Autodesk Inventor part; units mm, degrees
ref_plane "YZ Plane" through (0, 0, 0) normal (1, 0, 0) x (0, 1, 0)
ref_plane "XZ Plane" through (0, 0, 0) normal (0, 1, 0) x (-1, 0, 0)
ref_plane "XY Plane" through (0, 0, 0) normal (0, 0, 1) x (1, 0, 0)
sketch "スケッチ1" plane through (0, 0, 0) normal (0, 0, 1) x (1, 0, 0)
  line L0 (0, 0) -> (-26, 0)
  line L1 (0, 0) -> (-13, -73.8647)
  line L2 (-13, -73.8647) -> (-26, 0)
  dimension "d0" = 26
  dimension "d1" = 75
extrude "押し出し1" add sketch "スケッチ1" along normal mid plane 18
sketch "スケッチ2" plane through (0, 0, 9) normal (0, 0, 1) x (1, 0, 0)
  line L0 (-26, 0) -> (0, 0)
  line L1 (-2, 0) -> (-24, 0)
  line L2 (-2, 0) -> (-12.9991, -62.5063)
  line L3 (-2, 0) -> (61.4667, 0) construction
  line L4 (-12.9991, -62.5063) -> (-24, 0)
  line L5 (-13, -73.8647) -> (-26, 0)
  point P0 (-15.5606, -59.3154)
  dimension "d5" = 22
  dimension "d6" = 99.98
extrude "押し出し2" cut sketch "スケッチ2" against normal blind 20
fillet "フィレット2" radius 1 1 edges at (-12.9991, -62.5063, 0)
fillet "フィレット3" radius 2.6 1 edges at (-13, -73.8647, 0)
sketch "スケッチ3" plane through (0, 0, 9) normal (0, 0, 1) x (1, 0, 0)
  line L0 (-12.0143, -56.9099) -> (-2, 0)
  line L1 (-2.7039, -4) -> (-23.296, -4)
  line L2 (-13.984, -56.9099) -> (-24, 0)
  line L3 (-23.296, -4) -> (-23.296, -5)
  line L4 (-23.296, -5) -> (-2.7039, -5)
  line L5 (-2.7039, -5) -> (-2.7039, -4)
  point P0 (0, 0)
  point P1 (-23.12, -5)
  point P2 (-2.8798, -5)
  dimension "d11" = 1
extrude "押し出し3" add sketch "スケッチ3" against normal blind 18 contours L4 L2 L1 L0
sketch "スケッチ4" plane through (0, 0, 9) normal (0, 0, 1) x (1, 0, 0)
  line L0 (-3.119, -13.78) -> (-22.8808, -13.78)
  line L1 (-22.8808, -13.78) -> (-22.8808, -12.78)
  line L2 (-22.8808, -12.78) -> (-3.119, -12.78)
  line L3 (-3.119, -12.78) -> (-3.119, -13.78)
  line L4 (-3.119, -13.78) -> (-22.8808, -12.78) construction
  line L5 (-22.8808, -13.78) -> (-3.119, -12.78) construction
  line L6 (-5.0044, -22.56) -> (-20.9954, -22.56)
  line L7 (-20.9954, -22.56) -> (-20.9954, -21.56)
  line L8 (-20.9954, -21.56) -> (-5.0044, -21.56)
  line L9 (-5.0044, -21.56) -> (-5.0044, -22.56)
  line L10 (-5.0044, -22.56) -> (-20.9954, -21.56) construction
  line L11 (-20.9954, -22.56) -> (-5.0044, -21.56) construction
  line L12 (-6.4483, -31.34) -> (-19.5515, -31.34)
  line L13 (-19.5515, -31.34) -> (-19.5515, -30.34)
  line L14 (-19.5515, -30.34) -> (-6.4483, -30.34)
  line L15 (-6.4483, -30.34) -> (-6.4483, -31.34)
  line L16 (-6.4483, -31.34) -> (-19.5515, -30.34) construction
  line L17 (-19.5515, -31.34) -> (-6.4483, -30.34) construction
  line L18 (-7.4478, -40.12) -> (-18.552, -40.12)
  line L19 (-18.552, -40.12) -> (-18.552, -39.12)
  line L20 (-18.552, -39.12) -> (-7.4478, -39.12)
  line L21 (-7.4478, -39.12) -> (-7.4478, -40.12)
  line L22 (-7.4478, -40.12) -> (-18.552, -39.12) construction
  line L23 (-18.552, -40.12) -> (-7.4478, -39.12) construction
  line L24 (-9.5376, -48.9) -> (-16.4622, -48.9)
  line L25 (-16.4622, -48.9) -> (-16.4622, -47.9)
  line L26 (-16.4622, -47.9) -> (-9.5376, -47.9)
  line L27 (-9.5376, -47.9) -> (-9.5376, -48.9)
  line L28 (-9.5376, -48.9) -> (-16.4622, -47.9) construction
  line L29 (-16.4622, -48.9) -> (-9.5376, -47.9) construction
  point P0 (0, 0)
  point P1 (-12.9999, -13.28)
  point P2 (-12.9999, -22.06)
  point P3 (-12.9999, -30.84)
  point P4 (-12.9999, -39.62)
  point P5 (-12.9999, -48.4)
  dimension "d14" = 1
  dimension "d15" = 1
  dimension "d16" = 1
  dimension "d17" = 1
  dimension "d18" = 1
extrude "押し出し4" add sketch "スケッチ4" against normal blind 18
sketch "スケッチ5" plane through (0, 0, 0) normal (1, 0, 0) x (0, 1, 0)
  line L0 (-61.4647, -9) -> (-61.4647, 9)
  line L1 (-61.4647, 5.9) -> (-61.4647, 9)
  line L2 (0, 9) -> (-59.3154, 9)
  line L3 (-61.4647, 5.9) -> (0, 9)
  line L4 (0, 9) -> (-61.4647, 9)
  line L5 (-59.3154, -9) -> (-61.4647, -9)
  line L6 (-61.4647, -5.9) -> (-61.4647, -9)
  line L7 (-61.4647, -9) -> (0, -9)
  line L8 (0, -9) -> (-61.4647, -5.9)
  point P0 (0, 0)
extrude "押し出し5" cut sketch "スケッチ5" against normal blind 30
properties part number "finley_gripper_60"
CAD build for the part. Positions are in the model's coordinates, mm. A direction names the side the tool comes from. Coordinates: 2 decimals unless noted, no trailing zeros. Order: outer loops, then holes, each group sorted by start corner. A loop starts at its lowest first (then second) coordinate and runs counter-clockwise, first axis right, second up.
(1) Saw through at B-B, the plane x = -19.25. Write the cut outline in (y, z) (3 decimals).
Solution:
outline: (-38.353, -7.066) - (-26.989, -7.639) - (-26.989, 7.639) - (-38.353, 7.066) - close; (-22.56, -7.862) - (-21.56, -7.913) - (-21.56, 7.913) - (-22.56, 7.862) - close; (-13.78, -8.305) - (-12.78, -8.355) - (-12.78, 8.355) - (-13.78, 8.305) - close; (-5, -8.748) - (-4, -8.798) - (-4, 8.798) - (-5, 8.748) - close
(2) Saw through at C-C, the plane z = 3.5. Count the separate pieces of the cut face and the enclosed holes in it, and give its area (3 significant figures).
Solution:
separate pieces: 1
enclosed holes: 6
area: 324 mm2
(3) Drill centre lines: L1, parallel to Y at x = -16.5, z = -7.25; L2, parallel to X at y = -44.5, z = 1.75; L3, parallel to X at y = -54.5, z = -5.75. Where is each one in solid material? Low to high.
Solution:
L1: y = -31.34 to -30.34, -22.56 to -21.56, -13.78 to -12.78, -5 to -4
L2: x = -18.17 to -16.17, -9.83 to -7.83
L3: x = -16.41 to -14.41, -11.59 to -9.59
(4) Mould opens along Y. For faces 4 (the face through (-1, 0, 0)), 5 (the face through (-11.976, -30.589, -7.457)), 6 (the face through (-13, -13.78, 0)) say: released by +Y, released by -Y, zero draft, split by the parting line, or undercut.
Solution:
face 4: released by +Y
face 5: released by -Y
face 6: undercut
(5) Saw through at A-A, the plane y = -15.5. Write the cut outline in (x, z).
Solution:
outline: (-23.27, -8.22) - (-21.27, -8.22) - (-21.27, 8.22) - (-23.27, 8.22) - close; (-4.73, -8.22) - (-2.73, -8.22) - (-2.73, 8.22) - (-4.73, 8.22) - close
(6) Saw through at D-D, the plane x = -16.25. Write the cut outline in (y, z) (3 decimals).
Solution:
outline: (-55.399, -6.206) - (-44.035, -6.779) - (-44.035, 6.779) - (-55.399, 6.206) - close; (-40.12, -6.977) - (-39.12, -7.027) - (-39.12, 7.027) - (-40.12, 6.977) - close; (-31.34, -7.419) - (-30.34, -7.47) - (-30.34, 7.47) - (-31.34, 7.419) - close; (-22.56, -7.862) - (-21.56, -7.913) - (-21.56, 7.913) - (-22.56, 7.862) - close; (-13.78, -8.305) - (-12.78, -8.355) - (-12.78, 8.355) - (-13.78, 8.305) - close; (-5, -8.748) - (-4, -8.798) - (-4, 8.798) - (-5, 8.748) - close
(7) Which spindle directions (+Z, -Z, +X, -X, +Y, -Y) get a long thin tool onto all of the face, cutting with end or side? Do faces 1 (the face through (-23.643, -2.028, 0.126)), 2 (the face through (-20.707, -30.073, -0.126)), 3 (the face through (-20.88, -17.72, 0.12)). Say none if no direction does.
Solution:
face 1: +Z, -Z, +Y
face 2: +Z, -Z, -X, -Y
face 3: +Z, -Z
(8) Pin check, flat tips, straight feed: pin 1 Ø4 at (x, z) = (-12.5, -2.5) entering from +Y; pin 2 Ø1 at (x, y) = (-9, -15.5) entering from -Z; pin 3 Ø4 at (y, z) = (-20.5, -2) entering from -X; pin 4 Ø4 at (x, z) = (-9.5, -2) entering from -Y. Stop position of each tip, or through.
Solution:
pin 1: stops at y = -4
pin 2: passes through
pin 3: stops at x = -22.74
pin 4: stops at y = -60.99
